from build123d import *

# Parameters (mm, degrees)
SKETCH2_R           = 0.75
BOSS_EXTRUDE1_DEPTH = 12
FILLET1_R           = 0.75
FILLET2_R           = 1


with BuildPart() as part:
    # Sketch1 → Revolve1 (revolve)
    with BuildSketch(Plane.XY, mode=Mode.PRIVATE) as revolve1_sk:
        Polygon((0, 0), (9, 0), (9, 2.5), (6, 2.5), (6, 15), (5, 15), (5, 3), (0, 3), align=None)
    revolve(revolve1_sk.sketch.rotate(Axis((0, 0, 0), (0, 1, 0)), 90), axis=Axis((0, 0, 0), (0, 1, 0)))

    # Sketch2 → Boss-Extrude1 (add)
    with BuildSketch(Plane(origin=(0, 3, 0), x_dir=(1, 0, 0), z_dir=(0, 1, 0))):
        with Locations(Location((1.5, 2.5, 0), (0, 0, 270))):
            Circle(SKETCH2_R)
        with Locations(Location((1.5, -2.5, 0), (0, 0, 270))):
            Circle(SKETCH2_R)
        with Locations(Location((-2.5, 0, 0), (0, 0, 270))):
            Circle(SKETCH2_R)
    extrude(amount=BOSS_EXTRUDE1_DEPTH)

    # Fillet1
    fillet1_edges = [part.edges().sort_by_distance(p)[0] for p in [
        (1.5, 15, -3.25),
        (1.5, 15, 1.75),
        (-2.5, 15, -0.75),
    ]]
    fillet(fillet1_edges, radius=FILLET1_R)

    # Fillet2
    fillet2_edges = [part.edges().sort_by_distance(p)[0] for p in [
        (0, 2.5, 9),
    ]]
    fillet(fillet2_edges, radius=FILLET2_R)


solid = part.part
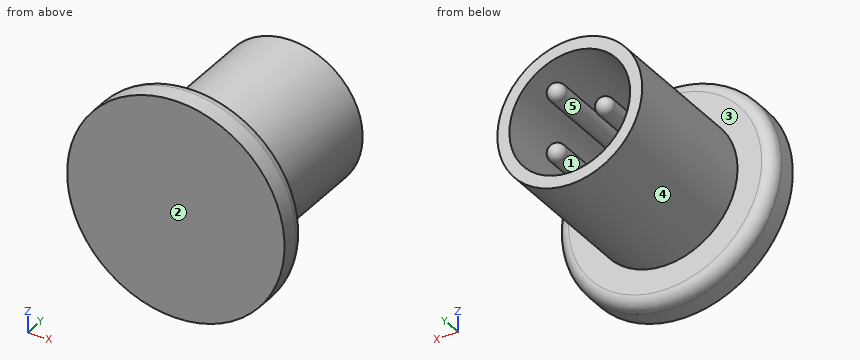
Geometry check sheet. Reference: the model listing, model coordinates, mm. Face numbers are marked on the shaded views. A direction names the side the tool comes from. Give positions to 0.01 mm unless a question says otherwise; leave off trailing zeros. Loops run counter-clockwise (first coordinate to the right, second up) from the corner with the lowest first, then second, coordinate; pieces in that order, holes last.
(1) Thickness scan on L1, parallel to X at y = 6, z = 0; L2, parallel to Z at x = -2.25, y = 3.5; L3, parallel to Y at x = 0, z = -1. Record the ranges inside material, lowest first.
From the geometry:
L1: x = -6 to -5, -3.25 to -1.75, 5 to 6
L2: z = -5.56 to -4.47, -0.71 to 0.71, 4.47 to 5.56
L3: y = 0 to 3
(2) Set-up check for the marked faces 1 and 2: record each of +Z, -Z, +X, -X, +Y, -Y from which the full face is reachable in a straight line by a thin tool's end or side.
From the geometry:
face 1: +Y
face 2: +Z, -Z, +X, -X, -Y
(3) Section check C-C on z = 0. Record the cut outline in (x, y).
From the geometry:
outline: (-9, 0) - (9, 0) - (9, 1.5) arc R1 ccw to (8, 2.5) - (6, 2.5) - (6, 15) - (5, 15) - (5, 3) - (-1.75, 3) - (-1.75, 14.25) arc R0.75 ccw to (-3.25, 14.25) - (-3.25, 3) - (-5, 3) - (-5, 15) - (-6, 15) - (-6, 2.5) - (-8, 2.5) arc R1 ccw to (-9, 1.5) - close
(4) Release check for a two-part mould opening along X. For the marked faces 3, 4 and 5 record: released by +X, released by -X, zero draft, split by the parting line, or undercut.
From the geometry:
face 3: zero draft
face 4: split by the parting line
face 5: undercut
(5) Section check A-A on y = 4. Record the cut outline in (x, z).
From the geometry:
outline: circle Ø12 at (0, 0); circle Ø1.5 at (-2.5, 0); circle Ø1.5 at (1.5, -2.5); circle Ø1.5 at (1.5, 2.5); hole circle Ø10 at (0, 0)
(6) Depth check by flat-ended pin: pin 1 Ø5 at (y, z) = (11, 3.5) entering from +X; pin 2 Ø6 at (x, y) = (6.5, 1.5) entering from +Z; pin 3 Ø3 at (y, z) = (10, -4.5) entering from -X. Enter the tip coordinate at first touch or a pass-through.
From the geometry:
pin 1: stops at x = 5.92
pin 2: stops at z = 8.29
pin 3: stops at x = -5.2
(7) Section check B-B on x = 0. Record the cut outline in (y, z), then the cut area to 3 significant figures.
From the geometry:
outline: (0, -9) - (1.5, -9) arc R1 ccw to (2.5, -8) - (2.5, -6) - (15, -6) - (15, -5) - (3, -5) - (3, 5) - (15, 5) - (15, 6) - (2.5, 6) - (2.5, 8) arc R1 ccw to (1.5, 9) - (0, 9) - close
area: 74.6 mm2
